Autodesk Inventor part; units mm, degrees
ref_plane "YZ Plane" through (0, 0, 0) normal (1, 0, 0) x (0, 1, 0)
ref_plane "XZ Plane" through (0, 0, 0) normal (0, 1, 0) x (-1, 0, 0)
ref_plane "XY Plane" through (0, 0, 0) normal (0, 0, 1) x (1, 0, 0)
sketch "草圖1" plane through (0, 0, 0) normal (1, 0, 0) x (0, 1, 0)
  line L0 (-22.5, -105) -> (22.5, -105)
  line L1 (22.5, -105) -> (22.5, 105)
  line L2 (22.5, 105) -> (-22.5, 105)
  line L3 (-22.5, 105) -> (-22.5, -105)
  line L4 (-22.5, -105) -> (22.5, 105) construction
  line L5 (22.5, -105) -> (-22.5, 105) construction
  point P0 (0, 0)
  dimension "d0" = 210
  dimension "d1" = 45
extrude "擠出1" add sketch "草圖1" along normal blind 25
fillet "圓角1" radius 22 4 edges at (12.5, 22.5, 105) (12.5, -22.5, 105) (12.5, 22.5, -105) (12.5, -22.5, -105)
sketch "草圖2" plane through (25, 0, 0) normal (1, 0, 0) x (0, 0, -1)
  line L0 (35, 6) -> (95, 6)
  line L1 (95, 6) -> (95, -6)
  line L2 (35, -6) -> (35, 6)
  line L3 (71, -6) -> (71, -22.5)
  line L4 (71, -22.5) -> (59, -22.5)
  line L5 (59, -22.5) -> (59, -6)
  line L6 (0, 0) -> (51.0559, 0) construction
  line L7 (95, -6) -> (71, -6)
  line L8 (59, -6) -> (35, -6)
  line L9 (65, -22.5) -> (65, 6) construction
  line L10 (-83, -22.5) -> (83, -22.5) construction
  line L11 (105, -0.5) -> (105, 0.5)
  dimension "d5" = 12
  dimension "d6" = 60
  dimension "d7" = 12
  dimension "d8" = 10
extrude "擠出2" cut sketch "草圖2" against normal blind 25
fillet "圓角2" radius 1 4 edges at (12.5, 6, -35) (12.5, -6, -35) (12.5, 6, -95) (12.5, -6, -95)
fillet "圓角3" radius 2 2 edges at (12.5, -6, -59) (12.5, -6, -71)
sketch "草圖3" plane through (0, 0, 0) normal (0, 1, 0) x (-1, 0, 0)
  line L0 (-25, 94) -> (-25, 34)
  line L1 (-70, 79) -> (-25, 94)
  line L2 (-70, 49) -> (-25, 34)
  line L3 (-32, 74) -> (-70, 74)
  line L4 (-70, 54) -> (-32, 54)
  line L5 (-32, 54) -> (-32, 74)
  line L6 (-70, 49) -> (-70, 54)
  line L7 (-70, 74) -> (-70, 79)
  line L8 (-32, 64) -> (-25, 64) construction
  line L9 (-25, 83) -> (-25, -59) construction
  line L10 (0, -59) -> (-25, -59)
  point P0 (0, 0)
  dimension "d13" = 113
  dimension "d14" = 20
  dimension "d15" = 5
  dimension "d16" = 20
  dimension "d17" = 45
  dimension "d21" = 38
extrude "擠出3" add sketch "草圖3" along normal mid plane 31
sketch "草圖4" plane through (0, -15.5, 0) normal (0, -1, 0) x (1, 0, 0)
  circle A0 centre (28.5, 69.95) radius 2
  circle A1 centre (28.5, 58.05) radius 2
  line L0 (25, 105) -> (25, 83) construction
  line L1 (70, 64) -> (28.5, 64) construction
  line L2 (70, 74) -> (32, 74) construction
  line L3 (32, 54) -> (70, 54) construction
  point P0 (0, 0)
  dimension "d22" = 3.5
  dimension "d23" = 4
  dimension "d24" = 11.9
  dimension "d25" = 10
extrude "擠出4" cut sketch "草圖4" against normal blind 31
properties part number "base"
Read the model definition and answer for the solid it produces. Units are mm, in the model's axes. A direction names the side the tool comes from. Coordinates: 2 decimals unless noted, no trailing zeros. Loops run counter-clockwise (first coordinate to the right, second up) from the corner with the lowest first, then second, coordinate; pieces in that order, holes last. Notation, with made-up numbers: (89, 43) -> (131, 43) arc R37 ccw to (131, 81) -> close; hole circle Ø1 at (4.5, -37.75). An arc over 180 degrees is marked (long way). Return JSON: item names as keys, results as strings.
Item 1: Find section D-D (x = 13). Determine the outline of the cut face in (y, z), plus the area to 3 significant figures.
Answers:
{"outline": "(-22.5, -83) arc R22 ccw to (-0.5, -105) -> (0.5, -105) arc R22 ccw to (22.5, -83) -> (22.5, 83) arc R22 ccw to (0.5, 105) -> (-0.5, 105) arc R22 ccw to (-22.5, 83) -> (-22.5, -59) -> (-8, -59) arc R2 ccw to (-6, -57) -> (-6, -36) arc R1 cw to (-5, -35) -> (5, -35) arc R1 cw to (6, -36) -> (6, -94) arc R1 cw to (5, -95) -> (-5, -95) arc R1 cw to (-6, -94) -> (-6, -73) arc R2 ccw to (-8, -71) -> (-22.5, -71) -> close", "area": "8,120 mm2"}
Item 2: For a pull along X with two mould halves and no side action, classify faces 1 (the cylindrical face through (28.24, -0.217, 60.033)), 2 (the flat face through (32, 0, 64)), 3 (the flat face through (0, 0, 1)), 4 (the flat face through (12, -22.5, -77)) as +X half, -X half, draft (parallel to the pull), parting line (faces both ways), or undercut.
Answers:
{"face 1": "undercut", "face 2": "+X half", "face 3": "-X half", "face 4": "draft"}
Item 3: Find section B-B (y = -10.5). Determine the outline of the cut face in (x, z).
Answers:
{"outline": "(0, -102.6) -> (25, -102.6) -> (25, -71) -> (0, -71) -> close; (0, -59) -> (25, -59) -> (25, 34) -> (70, 49) -> (70, 54) -> (32, 54) -> (32, 74) -> (70, 74) -> (70, 79) -> (25, 94) -> (25, 102.6) -> (0, 102.6) -> close; hole circle Ø4 at (28.5, 58.05); hole circle Ø4 at (28.5, 69.95)"}
Item 4: Flat-ended cylindrical pins translate along their axes: P1, Ø3, axis at x = 28.5, z = 58.05, coming from the -Y side; P2, Ø12, axis at x = 23, y = -10, coming from the +Z side; P3, Ø6, axis at y = 1, z = 67.5, coming from the +X side; P4, Ø4.5, axis at x = 16, y = -12, coming from the +Z side. Find the tip coordinate at first contact, or state that the pin passes through.
Answers:
{"P1": "passes through", "P2": "stops at z = 104.72", "P3": "stops at x = 32", "P4": "stops at z = 102.96"}
Item 5: Find section C-C (z = 69.95). Determine the outline of the cut face in (x, y).
Answers:
{"outline": "(0, -22.5) -> (25, -22.5) -> (25, -15.5) -> (26.5, -15.5) -> (26.5, 15.5) -> (25, 15.5) -> (25, 22.5) -> (0, 22.5) -> close; (30.5, -15.5) -> (32, -15.5) -> (32, 15.5) -> (30.5, 15.5) -> close"}
Item 6: Find the intervals of material crossed by probe 1 along Z at (x, y) = (28, -6); probe 2 along X at (y, z) = (-14, 27.5); probe 3 along Y at (x, z) = (18, -53.5), in increasing order.
Answers:
{"probe 1": "z = 35 to 56.11, 59.99 to 68.01, 71.89 to 93", "probe 2": "x = 0 to 25", "probe 3": "y = -22.5 to -6, 6 to 22.5"}
Item 7: Find section A-A (x = 46). Determine the outline of the cut face in (y, z).
Answers:
{"outline": "(-15.5, 41) -> (15.5, 41) -> (15.5, 54) -> (-15.5, 54) -> close; (-15.5, 74) -> (15.5, 74) -> (15.5, 87) -> (-15.5, 87) -> close"}
Item 8: For faces 5 (the flat face through (51, 0, 54)), 6 (the flat face through (43, 15.5, 78)), 7 (the flat face through (13, 0, -35)), 8 (the flat face through (43, -15.5, 78)), determine the directions among +Z, -Z, +X, -X, +Y, -Y from which every point of the face is accessible in a straight line to the end or side of a thin tool.
Answers:
{"face 5": "+X, +Y, -Y", "face 6": "+Z, -Z, +X, +Y", "face 7": "+X, -X", "face 8": "+Z, -Z, +X, -Y"}
